Model file for the job. Use its own axes, mm. Face numbers are marked on the shaded views. A direction names the side the tool comes from. Round coordinates to 2 decimals unless told otherwise and drop trailing zeros. Order: outer loops, then holes, each group sorted by start corner. A loop starts at its lowest first (then second) coordinate and runs counter-clockwise, first axis right, second up. Notation, with made-up numbers: (-32.5, -33.75) -> (10.5, -33.75) arc R28 ccw to (10.5, -14.75) -> close; hole circle Ø11 at (86.25, 7). An arc over 180 degrees is marked (long way). Answer as CSV lines item,"result".
Autodesk Inventor part; units mm, degrees
ref_plane "YZ Plane" through (0, 0, 0) normal (1, 0, 0) x (0, 1, 0)
ref_plane "XZ Plane" through (0, 0, 0) normal (0, 1, 0) x (-1, 0, 0)
ref_plane "XY Plane" through (0, 0, 0) normal (0, 0, 1) x (1, 0, 0)
sketch "Sketch1" plane through (0, 0, 0) normal (0, 1, 0) x (-1, 0, 0)
  line L0 (12, 21.5) -> (-12, 21.5)
  line L1 (-12, 21.5) -> (-12, -21.5)
  line L2 (-12, -21.5) -> (12, -21.5)
  line L3 (12, -21.5) -> (12, 21.5)
  line L4 (12.5, 22) -> (-12.5, 22)
  line L5 (-12.5, 22) -> (-12.5, -22)
  line L6 (-12.5, -22) -> (12.5, -22)
  line L7 (12.5, -22) -> (12.5, 22)
  line L8 (14.5, 24) -> (-14.5, 24)
  line L9 (-14.5, 24) -> (-14.5, -24)
  line L10 (-14.5, -24) -> (14.5, -24)
  line L11 (14.5, -24) -> (14.5, 24)
  circle A0 centre (8, 17.5) radius 1.6
  circle A1 centre (8, -17.5) radius 1.6
  circle A2 centre (-8, 17.5) radius 1.6
  circle A3 centre (-8, -17.5) radius 1.6
  line L12 (12, -13.5) -> (-12, -13.5)
  line L13 (12, 13.5) -> (-12, 13.5)
  point P0 (0, 0)
  dimension "d0" = 43
  dimension "d1" = 24
  dimension "d2" = 12
  dimension "d3" = 21.5
  dimension "d4" = 4
  dimension "d5" = 4
  dimension "d6" = 4
  dimension "d7" = 4
  dimension "d8" = 0.5
  dimension "d9" = 2
  dimension "d10" = 3.2
  dimension "d11" = 3.2
  dimension "d12" = 3.2
  dimension "d13" = 3.2
  dimension "d45" = 8
  dimension "d46" = 8
extrude "Extrusion1" add sketch "Sketch1" against normal blind 3 contours L3 L13 L1 L0 | L3 L12 L1 L13 | L3 L2 L1 L12 | L7 L6 L5 L4 | L11 L10 L9 L8 | A0 | A1 | A2 | A3
extrude "Extrusion3" cut sketch "Sketch1" against normal blind 6 contours A0 | A1 | A2 | A3
extrude "Extrusion7" add sketch "Sketch1" along normal blind 5.35 contours L3 L13 L1 L0 | L3 L2 L1 L12
fillet "Fillet3" radius 2 4 edges at (14.5, -1.5, 24) (-14.5, -1.5, 24) (14.5, -1.5, -24) (-14.5, -1.5, -24)
fillet "Fillet4" radius 2 8 edges at (12, 2.675, 21.5) (12, 2.675, 13.5) (-12, 2.675, 21.5) (-12, 2.675, 13.5) (12, 2.675, -13.5) (12, 2.675, -21.5) (-12, 2.675, -21.5) (-12, 2.675, -13.5)
equation "\"d10\" = d13"
equation "\"d11\" = d13"
equation "\"d12\" = d13"
properties part number "3DP_ASA_Bias_Tee_Case_Top"
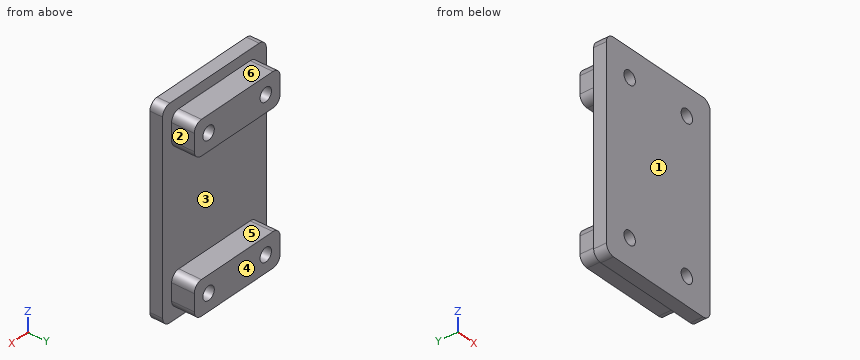
Q1. Wall check: L1, parallel to Z at x = 8, y = -0.5; L2, parallel to Z at x = 8, y = 5; L3, parallel to Z at x = 6.75, y = 2.75. Give the ranges that are in metal, low to high. Write a range as [from, to].
Checks:
L1,"[-24, -19.1], [-15.9, 15.9], [19.1, 24]"
L2,"[-21.5, -19.1], [-15.9, -13.5], [13.5, 15.9], [19.1, 21.5]"
L3,"[-21.5, -18.5], [-16.5, -13.5], [13.5, 16.5], [18.5, 21.5]"
Q2. Saw through at D-D (x = -3.25). Write the cut outline in (y, z).
Checks:
outline,"(-3, -24) -> (0, -24) -> (0, -21.5) -> (5.35, -21.5) -> (5.35, -13.5) -> (0, -13.5) -> (0, 13.5) -> (5.35, 13.5) -> (5.35, 21.5) -> (0, 21.5) -> (0, 24) -> (-3, 24) -> close"
Q3. Mould opens along Z. For the marked faces 3, 4, 5 and 6 say: +Z half, -Z half, draft (parallel to the pull), parting line (faces both ways), or undercut.
Checks:
face 3,"undercut"
face 4,"draft"
face 5,"undercut"
face 6,"+Z half"
Q4. Saw through at B-B (y = 1). Write the cut outline in (x, z).
Checks:
outline,"(-12, -19.5) arc R2 ccw to (-10, -21.5) -> (10, -21.5) arc R2 ccw to (12, -19.5) -> (12, -15.5) arc R2 ccw to (10, -13.5) -> (-10, -13.5) arc R2 ccw to (-12, -15.5) -> close; (-12, 15.5) arc R2 ccw to (-10, 13.5) -> (10, 13.5) arc R2 ccw to (12, 15.5) -> (12, 19.5) arc R2 ccw to (10, 21.5) -> (-10, 21.5) arc R2 ccw to (-12, 19.5) -> close; hole circle Ø3.2 at (-8, -17.5); hole circle Ø3.2 at (-8, 17.5); hole circle Ø3.2 at (8, -17.5); hole circle Ø3.2 at (8, 17.5)"
Q5. Saw through at A-A (x = -8). Write the cut outline in (y, z).
Checks:
outline,"(-3, -24) -> (0, -24) -> (0, -21.5) -> (5.35, -21.5) -> (5.35, -19.1) -> (-3, -19.1) -> close; (-3, -15.9) -> (5.35, -15.9) -> (5.35, -13.5) -> (0, -13.5) -> (0, 13.5) -> (5.35, 13.5) -> (5.35, 15.9) -> (-3, 15.9) -> close; (-3, 19.1) -> (5.35, 19.1) -> (5.35, 21.5) -> (0, 21.5) -> (0, 24) -> (-3, 24) -> close"
Q6. Saw through at C-C (z = -17.5). Write the cut outline in (x, y), plus the area to 3 significant figures.
Checks:
outline,"(-14.5, -3) -> (-9.6, -3) -> (-9.6, 5.35) -> (-12, 5.35) -> (-12, 0) -> (-14.5, 0) -> close; (-6.4, -3) -> (6.4, -3) -> (6.4, 5.35) -> (-6.4, 5.35) -> close; (9.6, -3) -> (14.5, -3) -> (14.5, 0) -> (12, 0) -> (12, 5.35) -> (9.6, 5.35) -> close"
area,"162 mm²"
Q7. Tool access for the marked faces 1 and 2: list every direction of +Z, -Z, +X, -X, +Y, -Y with a clear straight run to the whole face (end or side of a thin tool).
Checks:
face 1,"+Z, -Z, +X, -X, -Y"
face 2,"+Z, -Z, +X, +Y"
Q8. Flat gauge pins, fed straight in: pin 1 (2 mm diameter, centred on y = 2.5, z = -17, fed in from +X); pin 2 (3 mm diameter, centred on x = -8, z = 17.5, fed in from +Y); pin 3 (1.2 mm diameter, centred on y = 2.5, z = 17.5, fed in from -X); pin 4 (2.5 mm diameter, centred on x = 2.5, y = 3.5, fed in from -Z). Where does each tip first touch, or does it go through?
Checks:
pin 1,"x = 12"
pin 2,"through"
pin 3,"x = -12"
pin 4,"z = -21.5"
